Autodesk Inventor part; units mm, degrees
ref_plane "YZ Plane" through (0, 0, 0) normal (1, 0, 0) x (0, 1, 0)
ref_plane "XZ Plane" through (0, 0, 0) normal (0, 1, 0) x (-1, 0, 0)
ref_plane "XY Plane" through (0, 0, 0) normal (0, 0, 1) x (1, 0, 0)
ref_plane "Work Plane1" through (0, 0, 0) normal (0, 0, 1) x (1, 0, 0)
sketch "Sketch1" plane through (0, 0, 0) normal (0, 0, 1) x (1, 0, 0)
  circle A0 centre (7, -8.8957) radius 4
  circle A1 centre (-2.136, 8.8957) radius 4 construction
  line L0 (-8.905, 18.405) -> (-8.905, 11.3957) construction
  line L1 (-8.905, 11.3957) -> (-14.905, 11.3957) construction
  line L2 (-14.905, 11.3957) -> (-14.905, 6.3957) construction
  line L3 (-14.905, 6.3957) -> (-8.905, 6.3957) construction
  line L4 (-8.905, 6.3957) -> (-8.905, -6.3957) construction
  line L5 (-8.905, -6.3957) -> (-14.905, -6.3957) construction
  line L6 (-14.905, -6.3957) -> (-14.905, -11.3957) construction
  line L7 (-14.905, -11.3957) -> (-8.905, -11.3957) construction
  line L8 (-8.905, -11.3957) -> (-8.905, -18.405) construction
  line L9 (-8.905, -18.405) -> (15, -18.405) construction
  circle A2 centre (15, -16.5) radius 1.905 construction
  line L10 (15, -18.405) -> (34, -18.405) construction
  line L11 (34, 18.405) -> (34, -18.405) construction
  line L12 (34, 18.405) -> (15, 18.405) construction
  circle A3 centre (15, 16.5) radius 1.905 construction
  line L13 (15, 18.405) -> (-8.905, 18.405) construction
  arc A4 (13.5995, 17.7914) -> (16.4005, 17.7914) centre (15, 16.5) ccw construction
  line L14 (13.5995, 17.7914) -> (-8.705, 17.7914) construction
  line L15 (-8.705, 17.7914) -> (-8.705, 11.1957) construction
  line L16 (-8.705, 11.1957) -> (-14.705, 11.1957) construction
  line L17 (-14.705, 11.1957) -> (-14.705, 6.5957) construction
  line L18 (-14.705, 6.5957) -> (-8.705, 6.5957) construction
  line L19 (-8.705, 6.5957) -> (-8.705, 0) construction
  line L20 (-8.705, 0) -> (21.295, 0) construction
  line L21 (21.295, 0) -> (21.295, 17.7914) construction
  line L22 (21.295, 17.7914) -> (16.4005, 17.7914) construction
  circle A5 centre (-2.136, 8.8957) radius 4 construction
  circle A6 centre (7, -8.8957) radius 4 construction
  line L23 (-14.705, -11.1957) -> (-8.705, -11.1957)
  line L24 (-8.705, -11.1957) -> (-8.705, -6.5957)
  line L25 (-8.705, -6.5957) -> (-14.705, -6.5957)
  line L26 (-14.705, -6.5957) -> (-14.705, -11.1957)
  line L27 (-8.705, -17.7914) -> (21.295, -17.7914)
  line L28 (21.295, -17.7914) -> (21.295, 0)
  line L29 (21.295, 0) -> (-8.705, 0)
  line L30 (-8.705, 0) -> (-8.705, -17.7914)
  point P0 (0, 0)
  point P1 (-8.705, -8.8957)
  dimension "d0" = 0.2
extrude "Extrusion1" add sketch "Sketch1" along normal blind 15
sketch "Sketch2" plane through (0, 0, 15) normal (0, 0, 1) x (1, 0, 0)
  circle A0 centre (15, -16.5) radius 1.905
  point P0 (0, 0)
extrude "Extrusion2" cut sketch "Sketch2" against normal through all
sketch "Sketch3" plane through (21.295, -17.7914, 0) normal (1, 0, 0) x (0, 0, -1)
  line L0 (0, 0) -> (0, 17.7914) construction
  line L1 (0, 17.7914) -> (-15, 17.7914) construction
  line L2 (-15, 0) -> (-15, 17.7914) construction
  line L3 (0, 0) -> (-15, 0) construction
  line L4 (-18.5, 17.7914) -> (-28.5, 17.7914) construction
  line L5 (-18.5, 29.7914) -> (-18.5, 17.7914) construction
  line L6 (-28.5, 29.7914) -> (-18.5, 29.7914) construction
  line L7 (-28.5, 17.7914) -> (-28.5, 29.7914) construction
  line L8 (-2.5, 5.7914) -> (-12.5, 5.7914)
  line L9 (-12.5, 5.7914) -> (-12.5, 17.7914)
  line L10 (-12.5, 17.7914) -> (-2.5, 17.7914)
  line L11 (-2.5, 17.7914) -> (-2.5, 5.7914)
  point P0 (0, 17.7914)
  point P1 (-7.5, 17.7914)
extrude "Extrusion3" cut sketch "Sketch3" against normal blind 10
sketch "Sketch4" plane through (-8.705, 0, 0) normal (0, 1, 0) x (1, 0, 0)
  line L0 (30, -12.5) -> (20, -12.5)
  line L1 (20, -12.5) -> (20, -2.5)
  line L2 (20, -2.5) -> (30, -2.5)
  line L3 (30, 0) -> (30, -2.5)
  line L4 (30, 0) -> (0, 0)
  line L5 (0, 0) -> (0, -15)
  line L6 (30, -15) -> (0, -15)
  line L7 (30, -12.5) -> (30, -15)
  point P0 (8.705, 0)
extrude "Extrusion4" cut sketch "Sketch4" against normal blind 0.6
properties part number "long selector"
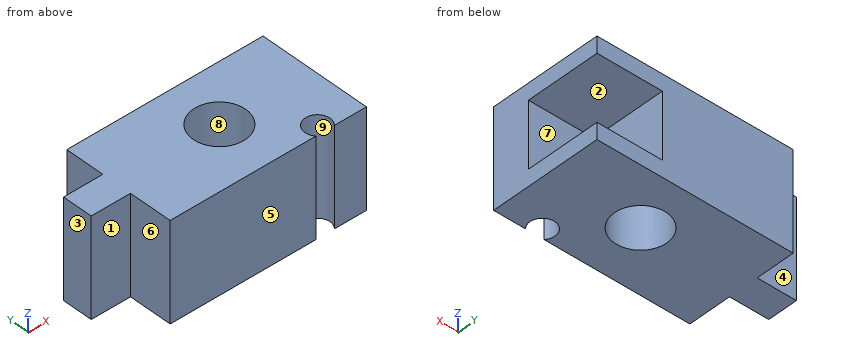
Part model, mm, in its own coordinate system. Face numbers are marked on the shaded views. A direction names the side the tool comes from. Round coordinates to 2 decimals unless told otherwise and drop trailing zeros. Loops run counter-clockwise (first coordinate to the right, second up) from the corner with the lowest first, then second, coordinate; pieces in that order, holes last. Notation, with made-up numbers: (3, 73.5) -> (40, 73.5) arc R20 cw to (40, 104.5) -> close; hole circle Ø6 at (31, -27). An arc over 180 degrees is marked (long way). Use a Markdown table: item, result.
1) Drop flat-ended pins along their axis: pin 1 Ø5 at (x, z) = (-12.5, 9) entering from -Y; pin 2 Ø3 at (y, z) = (-3, 4) entering from -X (3 decimals); pin 3 Ø5 at (y, z) = (-5.5, 9) entering from +X (3 decimals); pin 4 Ø5 at (x, y) = (7, -8.9) entering from +Z. Give the stop position or say it passes through.
The answers:
| item | result |
|---|---|
| pin 1 | stops at y = -11.2 |
| pin 2 | stops at x = -8.705 |
| pin 3 | stops at x = 11.295 |
| pin 4 | passes through |
2) Tool access for the marked faces 1, 2, 3, 4 and 5: list every direction of +Z, -Z, +X, -X, +Y, -Y with a clear straight run to the whole face (end or side of a thin tool).
The answers:
| item | result |
|---|---|
| face 1 | +Z, -Z, -X, -Y |
| face 2 | +X, +Y |
| face 3 | +Z, -Z, -X, +Y, -Y |
| face 4 | +Z, -Z, -X, +Y |
| face 5 | +Z, -Z, +X, -X, -Y |
3) Cut at B-B, the plane y = -16.5. List the corners of the cut face in (x, z) (3 decimals).
The answers:
| item | result |
|---|---|
| outline | (-8.705, 0) -> (13.095, 0) -> (13.095, 15) -> (-8.705, 15) -> close; (16.905, 0) -> (21.295, 0) -> (21.295, 15) -> (16.905, 15) -> close |
4) Probe line 1 (X direction, y = -9, z = 4.5) (3 decimals); line 2 (X direction, y = -8.75, z = 12.75) (3 decimals); line 3 (Y direction, x = 7, z = 3.75). List the from-to ranges inside material, lowest first. Write a range as [from, to].
The answers:
| item | result |
|---|---|
| line 1 | x = [-14.705, 3.001], [10.999, 11.295] |
| line 2 | x = [-14.705, 3.003], [10.997, 21.295] |
| line 3 | y = [-17.79, -12.9], [-4.9, -0.6] |
5) Cut at A-A, the plane x = 7. List the corners of the cut face in (y, z), and give its area (3 significant figures).
The answers:
| item | result |
|---|---|
| outline | (-17.79, 0) -> (-12.9, 0) -> (-12.9, 15) -> (-17.79, 15) -> close; (-4.9, 0) -> (-0.6, 0) -> (-0.6, 15) -> (-4.9, 15) -> close |
| area | 138 mm2 |
6) Cut at C-C, the plane z = 9. List the corners of the cut face in (x, y) (3 decimals), and give its area (3 significant figures).
The answers:
| item | result |
|---|---|
| outline | (-14.705, -11.196) -> (-8.705, -11.196) -> (-8.705, -17.791) -> (13.6, -17.791) arc R1.905 cw (long way) to (16.4, -17.791) -> (21.295, -17.791) -> (21.295, -12) -> (11.295, -12) -> (11.295, -0.6) -> (-8.705, -0.6) -> (-8.705, -6.596) -> (-14.705, -6.596) -> close; hole circle Ø8 at (7, -8.896) |
| area | 369 mm2 |
7) Cut at D-D, the plane x = 15. List the corners of the cut face in (y, z) (3 decimals).
The answers:
| item | result |
|---|---|
| outline | (-14.595, 0) -> (-0.6, 0) -> (-0.6, 2.5) -> (-12, 2.5) -> (-12, 12.5) -> (-0.6, 12.5) -> (-0.6, 15) -> (-14.595, 15) -> close |
8) Pull direction X, two halves, no side cores. Call the marked faces 6, 7, 8 and 9: pulls with the +X half, pulls with the -X half, needs draft (parallel to the pull), parting line crosses it, or undercut.
The answers:
| item | result |
|---|---|
| face 6 | pulls with the -X half |
| face 7 | needs draft |
| face 8 | undercut |
| face 9 | undercut |
